Design review of the part shown in the three views and the two pictorial views. Dimensions are in mm from the part's minimum x, y and z. A direction names the side the tool comes from. Round coordinates to 2 decimals unless told otherwise and drop trailing zeros. Loops run counter-clockwise (first coordinate to the right, second up) from the corner with the lowest first, then second, coordinate; pieces in that order, holes last. Notation, with made-up numbers: M -12.75,-25.75 L 17.25,-25.75 A21 ccw 17.25,-18.75 Z; hole C -0.5,40 d5. An arc over 180 degrees is marked long. Return JSON: item names as keys, results as strings. Group by question number.
Q1. To check wall thickness, follow line 1 along Z through (x, y) = (107.95, 33.75); line 2 along Y through (x, z) = (121, 10); line 3 along X through (y, z) = (8, 7). State the ranges of each line that lie inside material, in increasing order.
Q2. Consider section A-A (x = 107.95). State the section outline as (y, z) points, and give its area (3 significant figures).
Q3. Draft analysis for pull direction Z (two halves, no side actions). For the marked faces 1, 2 and 3, state which applies: pulls with the +Z half, pulls with the -Z half, needs draft (parallel to the pull), parting line crosses it, or undercut.
Q4. For the marked faces 4, 5 and 6, list the 3-axis set-ups (+Z, -Z, +X, -X, +Y, -Y) from which the entire face can be reached by the end or side of a thin tool; tool diameter is ignored.
Q5. Consider section D-D (y = 9.5). State the section outline as (x, z) points, and give its area (3 significant figures).
Q6. Clearance check with flat-ended pins moving along their axes: pin 1 Ø16 at (x, z) = (103, 22.5) entering from -Y; pin 2 Ø9.5 at (x, z) = (107.95, 16.61) entering from -Y; pin 3 Ø15 at (y, z) = (7, 12) entering from +X; pin 4 Ø9.5 at (x, y) = (117, 32) entering from +Z. State where each tip first meets the part, or that it passes through.
Q7. Consider section B-B (z = 10.5). State the section outline as (x, y) points.
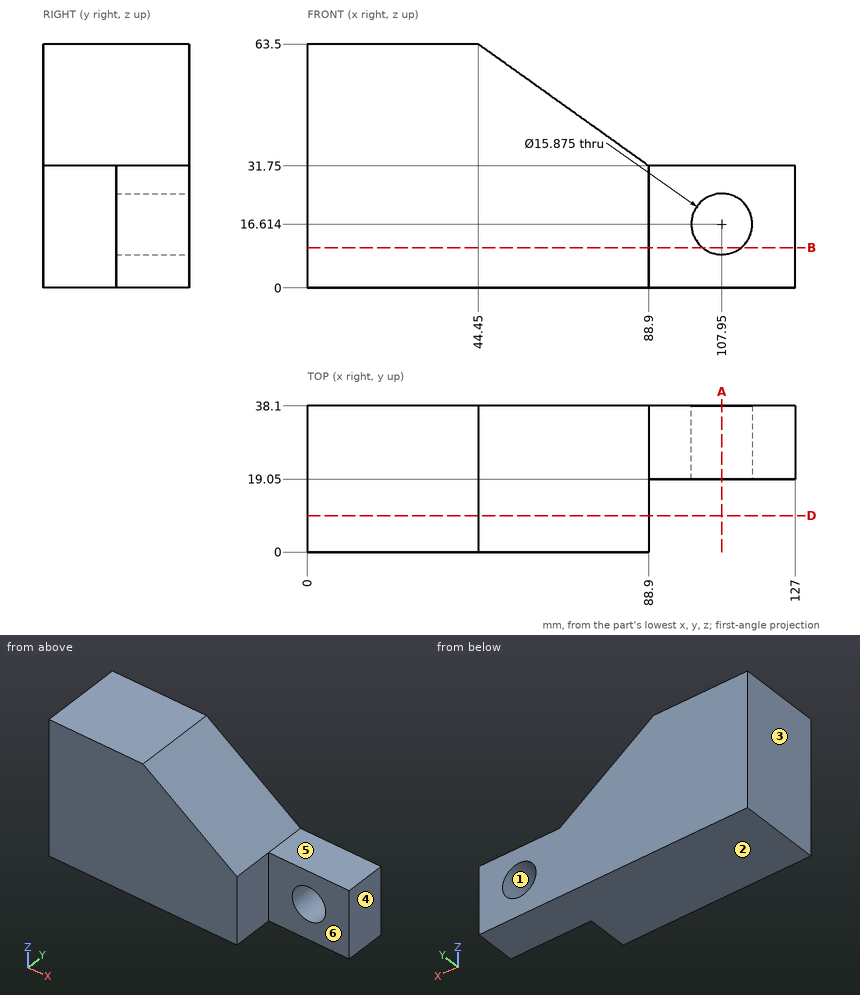
Values:
{
 "1": {"line 1": "z = 0 to 8.68, 24.55 to 31.75", "line 2": "y = 19.05 to 38.1", "line 3": "x = 0 to 88.9"},
 "2": {"outline": "M 19.05,0 L 38.1,0 L 38.1,8.68 L 19.05,8.68 Z; M 19.05,24.55 L 38.1,24.55 L 38.1,31.75 L 19.05,31.75 Z", "area": "302 mm2"},
 "3": {"face 1": "undercut", "face 2": "pulls with the -Z half", "face 3": "needs draft"},
 "4": {"face 4": "+Z, -Z, +X, +Y, -Y", "face 5": "+Z, +X, +Y, -Y", "face 6": "+Z, -Z, +X, -Y"},
 "5": {"outline": "M 0,0 L 88.9,0 L 88.9,31.75 L 44.45,63.5 L 0,63.5 Z", "area": "4,940 mm2"},
 "6": {"pin 1": "stops at y = 19.05", "pin 2": "passes through", "pin 3": "stops at x = 88.9", "pin 4": "stops at z = 31.75"},
 "7": {"outline": "M 0,0 L 88.9,0 L 88.9,19.05 L 102.89,19.05 L 102.89,38.1 L 0,38.1 Z; M 113.01,19.05 L 127,19.05 L 127,38.1 L 113.01,38.1 Z"}
}
